Could you check a few things on this model? Use its own coordinates, in mm. Face numbers are marked on the shaded views. Round coordinates to 2 decimals unless told otherwise and drop trailing zeros. Write each loop counter-clockwise with the first axis right and the second up, starting at its lowest first coordinate (ties: lowest second). Pieces come first, ordered by that corner, then holes.
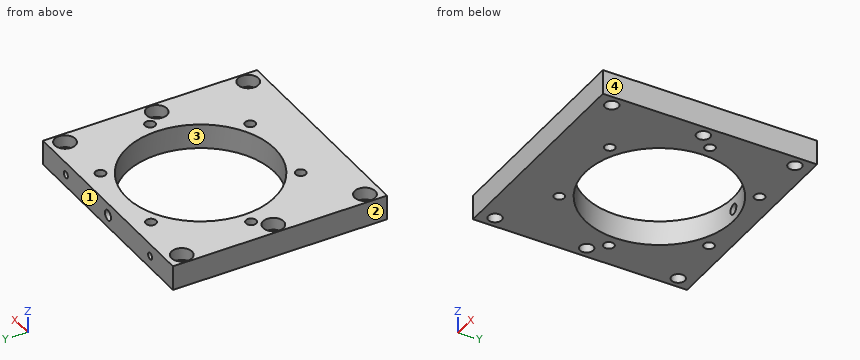
```python
from build123d import *

# Parameters (mm, degrees)
CROQUIS1_W                = 108
CROQUIS1_H                = 104
CROQUIS1_R                = 36
CROQUIS1_R_2              = 3.25
SALIENTE_EXTRUIR1_DEPTH   = 6
TALADRO_ROSCADO_M61_D     = 5
CROQUIS4_R                = 5
CORTAR_EXTRUIR1_DEPTH     = 6
TALADRO_ROSCADO_M62_D     = 5
TALADRO_ROSCADO_M62_DEPTH = 27
TALADRO_ROSCADO_M62_TIP   = 1.502151548
TALADRO_ROSCADO_M41_D     = 3.3
TALADRO_ROSCADO_M41_DEPTH = 12
TALADRO_ROSCADO_M41_TIP   = 0.991420021


with BuildPart() as part:
    # Croquis1 → Saliente-Extruir1 (new body, symmetric)
    with BuildSketch(Plane.XY):
        Rectangle(CROQUIS1_W, CROQUIS1_H)
        with Locations((0, 7)):
            Circle(CROQUIS1_R, mode=Mode.SUBTRACT)
        with Locations((-48.5, 44.5)):
            Circle(CROQUIS1_R_2, mode=Mode.SUBTRACT)
        with Locations((-48.5, 0)):
            Circle(CROQUIS1_R_2, mode=Mode.SUBTRACT)
        with Locations((-48.5, -44.5)):
            Circle(CROQUIS1_R_2, mode=Mode.SUBTRACT)
        with Locations((48.5, -44.5)):
            Circle(CROQUIS1_R_2, mode=Mode.SUBTRACT)
        with Locations((48.5, 0)):
            Circle(CROQUIS1_R_2, mode=Mode.SUBTRACT)
        with Locations((48.5, 44.5)):
            Circle(CROQUIS1_R_2, mode=Mode.SUBTRACT)
    extrude(amount=SALIENTE_EXTRUIR1_DEPTH, both=True)

    # Taladro roscado M61 (through all)
    with Locations(Plane.XY.offset(6)):
        with Locations((-21, 43.373066959), (-42, 7), (-21, -29.373066959), (21, -29.373066959), (42, 7), (21, 43.373066959)):
            Hole(TALADRO_ROSCADO_M61_D / 2)

    # Croquis4 → Cortar-Extruir1 (cut)
    with BuildSketch(Plane.XY.offset(6)):
        with Locations((-48.5, 44.5)):
            Circle(CROQUIS4_R)
        with Locations((-48.5, 0)):
            Circle(CROQUIS4_R)
        with Locations((-48.5, -44.5)):
            Circle(CROQUIS4_R)
        with Locations((48.5, -44.5)):
            Circle(CROQUIS4_R)
        with Locations((48.5, 0)):
            Circle(CROQUIS4_R)
        with Locations((48.5, 44.5)):
            Circle(CROQUIS4_R)
    extrude(amount=-CORTAR_EXTRUIR1_DEPTH, mode=Mode.SUBTRACT)

    # Taladro roscado M62
    with Locations(Plane(origin=(0, 52, 0), x_dir=(-1, 0, 0), z_dir=(0, 1, 0))):
        with Locations((0, 0)):
            Hole(TALADRO_ROSCADO_M62_D / 2, depth=TALADRO_ROSCADO_M62_DEPTH)
            with Locations((0, 0, -(TALADRO_ROSCADO_M62_DEPTH + TALADRO_ROSCADO_M62_TIP / 2))):  # 118° drill point
                Cone(0, TALADRO_ROSCADO_M62_D / 2, TALADRO_ROSCADO_M62_TIP, mode=Mode.SUBTRACT)

    # Taladro roscado M41
    with Locations(Plane(origin=(0, 52, 0), x_dir=(-1, 0, 0), z_dir=(0, 1, 0))):
        with Locations((35, 0), (-35, 0)):
            Hole(TALADRO_ROSCADO_M41_D / 2, depth=TALADRO_ROSCADO_M41_DEPTH)
            with Locations((0, 0, -(TALADRO_ROSCADO_M41_DEPTH + TALADRO_ROSCADO_M41_TIP / 2))):  # 118° drill point
                Cone(0, TALADRO_ROSCADO_M41_D / 2, TALADRO_ROSCADO_M41_TIP, mode=Mode.SUBTRACT)


solid = part.part
```
Q1. Imagine slicing it at B-B, the plane x = 0. Write out the boundary of the cut face in (y, z).
Q2. Imagine slicing it at D-D, the plane z = 4. Count the separate pieces of the cut face and the enclosed holes in it, then the cut area to 3 significant figures.
Q3. I'm going to push flat-ended pins straight in: pin 1 Ø2 at (x, z) = (35, 0) entering from +Y; pin 2 Ø13 at (x, y) = (48.5, -44.5) entering from +Z; pin 3 Ø8.5 at (x, y) = (-48.5, 44.5) entering from +Z. Where does each tip first touch, or does it pass through?
Q4. Imagine slicing it at C-C, the plane y = 34. Write out the boundary of the cut face in (x, z).
Q5. Imagine slicing it at A-A, the plane y = 7. Write out the boundary of the cut face in (x, z).
Q6. If I drill on L1, parallel to Y at x = 48.5, z = -2; L2, parallel to Y at x = -48.5, z = 4.1; L3, parallel to Z at x = 0, y = 49, over which ranges is the centre line in solid material (lowest first)?
Q7. We'd pull the mould along X, two halves only. Please class the marked faces 1, 2, 3 and 4: pulls with the +X half, pulls with the -X half, needs draft (parallel to the pull), parting line crosses it, or undercut.
Results found:
1. outline: (-52, -6) - (-29, -6) - (-29, 6) - (-52, 6) - close; (43, -6) - (52, -6) - (52, -2.5) - (43, -2.5) - close; (43, 2.5) - (52, 2.5) - (52, 6) - (43, 6) - close
2. separate pieces: 1
2. enclosed holes: 13
2. area: 6,570 mm2
3. pin 1: stops at y = 39.61
3. pin 2: stops at z = 6
3. pin 3: stops at z = 0
4. outline: (-54, -6) - (-23.81, -6) - (-23.81, 6) - (-54, 6) - close; (23.81, -6) - (54, -6) - (54, 6) - (23.81, 6) - close
5. outline: (-54, -6) - (-44.5, -6) - (-44.5, 6) - (-54, 6) - close; (-39.5, -6) - (-36, -6) - (-36, 6) - (-39.5, 6) - close; (36, -6) - (39.5, -6) - (39.5, 6) - (36, 6) - close; (44.5, -6) - (54, -6) - (54, 6) - (44.5, 6) - close
6. L1: y = -52 to -47.75, -41.25 to -3.25, 3.25 to 41.25, 47.75 to 52
6. L2: y = -52 to -49.5, -39.5 to -5, 5 to 39.5, 49.5 to 52
6. L3: z = -6 to -2.5, 2.5 to 6
7. face 1: needs draft
7. face 2: pulls with the -X half
7. face 3: undercut
7. face 4: pulls with the +X half
